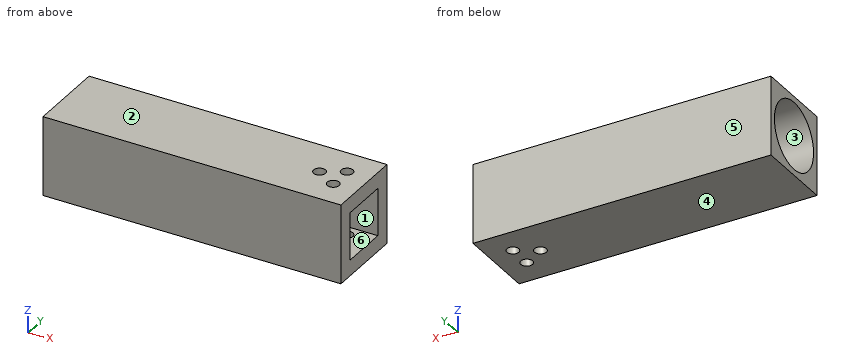
```python
from build123d import *

# Parameters (mm, degrees)
SKETCH1_W                       = 63.5
SKETCH1_H                       = 63.5
SKETCH1_W_2                     = 38.1
SKETCH1_H_2                     = 38.1
BOSS_EXTRUDE1_DEPTH             = 50.8
SKETCH5_W                       = 63.5
SKETCH5_H                       = 63.5
SKETCH5_R                       = 26.9875
BOSS_EXTRUDE2_DEPTH             = 187.8
F_97_0_375_DIAMETER_HOLE2_D     = 9.525
F_97_0_375_DIAMETER_HOLE2_DEPTH = 12.7
F_97_0_375_DIAMETER_HOLE3_D     = 9.525


with BuildPart() as part:
    # Sketch1 → Boss-Extrude1 (new body)
    with BuildSketch(Plane.YZ):
        Rectangle(SKETCH1_W, SKETCH1_H)
        Rectangle(SKETCH1_W_2, SKETCH1_H_2, mode=Mode.SUBTRACT)
    extrude(amount=BOSS_EXTRUDE1_DEPTH)

    # Sketch5 → Boss-Extrude2 (add)
    with BuildSketch(Plane.ZY):
        Rectangle(SKETCH5_W, SKETCH5_H)
        Circle(SKETCH5_R, mode=Mode.SUBTRACT)
    extrude(amount=BOSS_EXTRUDE2_DEPTH)

    # #97 (0.375) Diameter Hole2
    with Locations(Plane(origin=(0, 0, -31.75), x_dir=(-1, 0, 0), z_dir=(0, 0, -1))):
        with Locations((-15.252216058, 0), (-31.75, 9.525), (-31.75, -9.525)):
            Hole(F_97_0_375_DIAMETER_HOLE2_D / 2, depth=F_97_0_375_DIAMETER_HOLE2_DEPTH)

    # #97 (0.375) Diameter Hole3 (through all)
    with Locations(Plane.XY.offset(31.75)):
        with Locations((31.75, -9.525), (31.75, 9.525), (15.252216058, 0)):
            Hole(F_97_0_375_DIAMETER_HOLE3_D / 2)


solid = part.part
```
Geometry: final body of the model. Coordinates: model frame, mm. Face numbers are marked on the shaded views. A direction names the side the tool comes from. Round coordinates to 2 decimals unless told otherwise and drop trailing zeros. Order: outer loops, then holes, each group sorted by start corner. A loop starts at its lowest first (then second) coordinate and runs counter-clockwise, first axis right, second up. Notation, with made-up numbers: (23.5, 39.5) -> (50.5, 39.5) arc R10 ccw to (50.5, 43.5) -> close; hole circle Ø1 at (-35.75, 85). An arc over 180 degrees is marked (long way). Use one line per item in the form item = value. Start each with the question number.
1. Cut plane B-B (z = 0). Return the cut outline in (x, y), then the cut area to 3 significant figures.
2. Draft query along Y for the marked faces 3, 4, 5 and 6. Return one class per face: pulls with the +Y half, pulls with the -Y half, needs draft (parallel to the pull), parting line crosses it, or undercut.
3. Pin query (flat end, axial travel): pin 1 Ø8.5 at (x, y) = (31.75, 9.525) entering from -Z. Return the tip coordinate at first contact, or that it passes through.
4. Cut plane C-C (y = 0). Return the cut outline in (x, z).
5. Reachability of the marked faces 1 and 2 from +Z, -Z, +X, -X, +Y, -Y: full face, straight path, thin tool, end or side. Return the list, or none.
6. Line query: probe 1 along Y at (x, z) = (31.75, -28.25); probe 2 along Y at (x, z) = (31, -26); probe 3 along X at (y, z) = (-10, -20). Output: solid intervals per line, ascending.
7. Cut plane A-A (x = 31.75). Return the cut outline in (y, z).
Solution:
q1.outline = (-187.8, -31.75) -> (50.8, -31.75) -> (50.8, -19.05) -> (0, -19.05) -> (0, -26.99) -> (-187.8, -26.99) -> close; (-187.8, 26.99) -> (0, 26.99) -> (0, 19.05) -> (50.8, 19.05) -> (50.8, 31.75) -> (-187.8, 31.75) -> close
q1.area = 3,080 mm^2
q2.face_3 = undercut
q2.face_4 = needs draft
q2.face_5 = pulls with the +Y half
q2.face_6 = undercut
q3.pin_1 = through
q4.outline = (-187.8, -31.75) -> (10.49, -31.75) -> (10.49, -19.05) -> (0, -19.05) -> (0, -26.99) -> (-187.8, -26.99) -> close; (-187.8, 26.99) -> (0, 26.99) -> (0, 19.05) -> (10.49, 19.05) -> (10.49, 31.75) -> (-187.8, 31.75) -> close; (20.01, -31.75) -> (50.8, -31.75) -> (50.8, -19.05) -> (20.01, -19.05) -> close; (20.01, 19.05) -> (50.8, 19.05) -> (50.8, 31.75) -> (20.01, 31.75) -> close
q5.face_1 = +X, -X
q5.face_2 = +Z, +X, -X, +Y, -Y
q6.probe_1 = -31.75 to -14.29, -4.76 to 4.76, 14.29 to 31.75
q6.probe_2 = -31.75 to -14.23, -4.82 to 4.82, 14.23 to 31.75
q6.probe_3 = 0 to 27.01, 36.49 to 50.8
q7.outline = (-31.75, -31.75) -> (-14.29, -31.75) -> (-14.29, -19.05) -> (-19.05, -19.05) -> (-19.05, 19.05) -> (-14.29, 19.05) -> (-14.29, 31.75) -> (-31.75, 31.75) -> close; (-4.76, -31.75) -> (4.76, -31.75) -> (4.76, -19.05) -> (-4.76, -19.05) -> close; (-4.76, 19.05) -> (4.76, 19.05) -> (4.76, 31.75) -> (-4.76, 31.75) -> close; (14.29, -31.75) -> (31.75, -31.75) -> (31.75, 31.75) -> (14.29, 31.75) -> (14.29, 19.05) -> (19.05, 19.05) -> (19.05, -19.05) -> (14.29, -19.05) -> close
